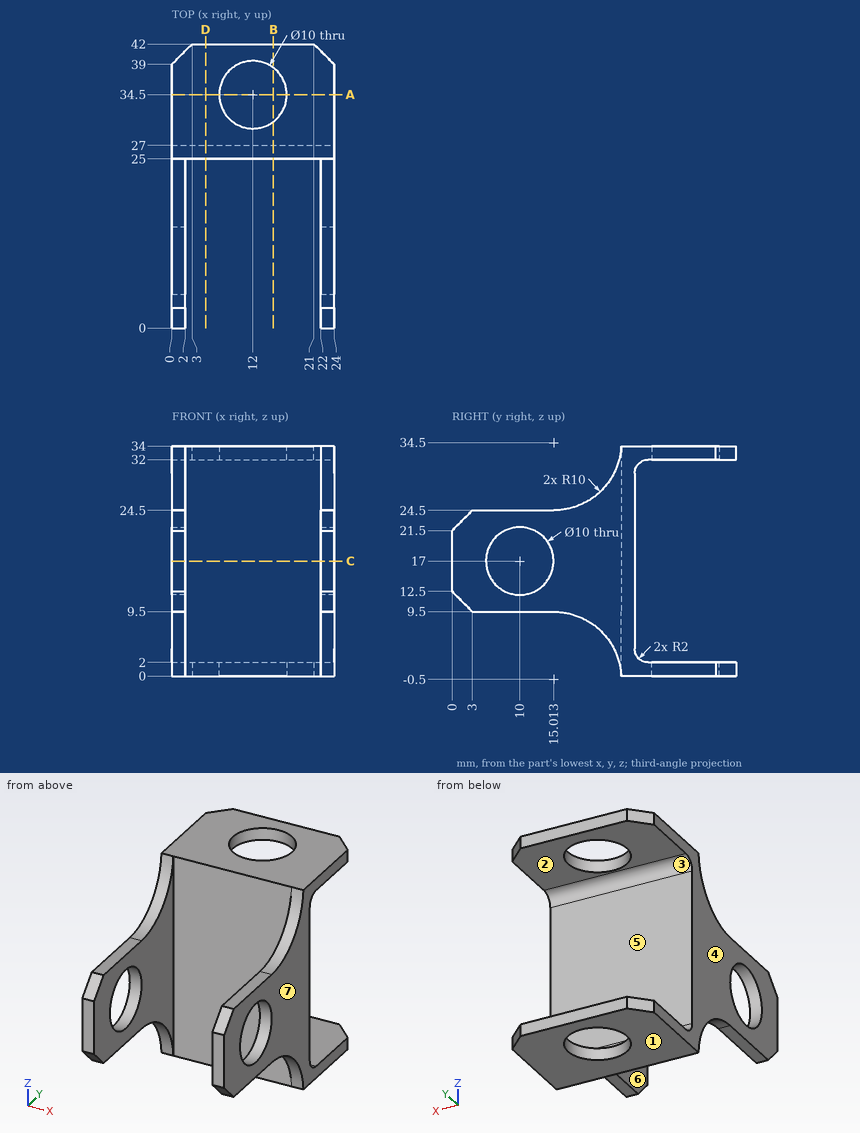
Could you check a few things on this drawing? It's one solid part, dimensions in mm from its lowest x, y, z. A direction names the side the tool comes from. Round coordinates to 2 decimals unless told otherwise and drop trailing zeros. Write each loop counter-clockwise with the first axis right and the second up, starting at its lowest first coordinate (ties: lowest second). Pieces come first, ordered by that corner, then holes. Notation, with made-up numbers: M 65.5,10.25 L 70.5,10.25 A3 cw 70.5,15.25 Z; hole C 2.5,9 d9. An arc over 180 degrees is marked long. Answer as CSV lines item,"result". Start each with the question number.
1. Suppose I cut it at C-C on z = 17. Write out the boundary of the cut face in (x, y), then the cut area to 3 significant figures.
2. On a 3-axis mill with a long thin cutter (end or side, diameter ignored), from which of +Z, -Z, +X, -X, +Y, -Y can I reach the whole of each face in a straight line? I mean the marked faces 5, 6 and 7. Say none if no direction works.
3. I'm going to push flat-ended pins straight in: pin 1 Ø2 at (x, y) = (1, 9.5) entering from -Z; pin 2 Ø6 at (x, y) = (16, 32.5) entering from +Z; pin 3 Ø12 at (x, z) = (8.5, 22.5) entering from +Y; pin 4 Ø4 at (x, y) = (10.5, 35) entering from -Z. Where does each tip first touch, or does it pass through?
4. Suppose I cut it at D-D on x = 5. Write out the boundary of the cut face in (y, z), then the cut area to 3 significant figures.
5. Thinking about a two-plate mould opening in Z: for the marked faces 1, 2, 3 and 4, which applies, released by +Z, released by -Z, zero draft, split by the parting line, or undercut?
6. Suppose I cut it at A-A on y = 34.5. Write out the boundary of the cut face in (x, z).
7. Suppose I cut it at B-B on x = 15. Write out the boundary of the cut face in (y, z).
8. I need wall thicknesses on probe 1 along Y at (x, z) = (22.4, 17); probe 2 along Y at (x, z) = (12, 0.85); probe 3 along Z at (x, y) = (22.75, 29.5). Which ranges of each line are inside material? Lowest first, please.
Check result:
1,outline,"M 0,0 L 2,0 L 2,5 L 0,5 Z; M 0,15 L 2,15 L 2,25 L 22,25 L 22,15 L 24,15 L 24,27 L 0,27 Z; M 22,0 L 24,0 L 24,5 L 22,5 Z"
1,area,"108 mm2"
2,face 5,"+X, -X, +Y"
2,face 6,"+Z, -Z, -Y"
2,face 7,"+Z, -Z, +X, +Y, -Y"
3,pin 1,"stops at z = 9.5"
3,pin 2,"stops at z = 34"
3,pin 3,"stops at y = 27"
3,pin 4,"passes through"
4,outline,"M 25,0 L 42,0 L 42,2 L 29,2 A2 cw 27,4 L 27,30 A2 cw 29,32 L 42,32 L 42,34 L 25,34 Z"
4,area,"130 mm2"
5,face 1,"released by -Z"
5,face 2,"undercut"
5,face 3,"undercut"
5,face 4,"zero draft"
6,outline,"M 0,0 L 7,0 L 7,2 L 0,2 Z; M 0,32 L 7,32 L 7,34 L 0,34 Z; M 17,0 L 24,0 L 24,2 L 17,2 Z; M 17,32 L 24,32 L 24,34 L 17,34 Z"
7,outline,"M 25,0 L 30.5,0 L 30.5,2 L 29,2 A2 cw 27,4 L 27,30 A2 cw 29,32 L 30.5,32 L 30.5,34 L 25,34 Z; M 38.5,0 L 42,0 L 42,2 L 38.5,2 Z; M 38.5,32 L 42,32 L 42,34 L 38.5,34 Z"
8,probe 1,"y = 0 to 5, 15 to 27"
8,probe 2,"y = 25 to 29.5, 39.5 to 42"
8,probe 3,"z = 0 to 2, 32 to 34"
